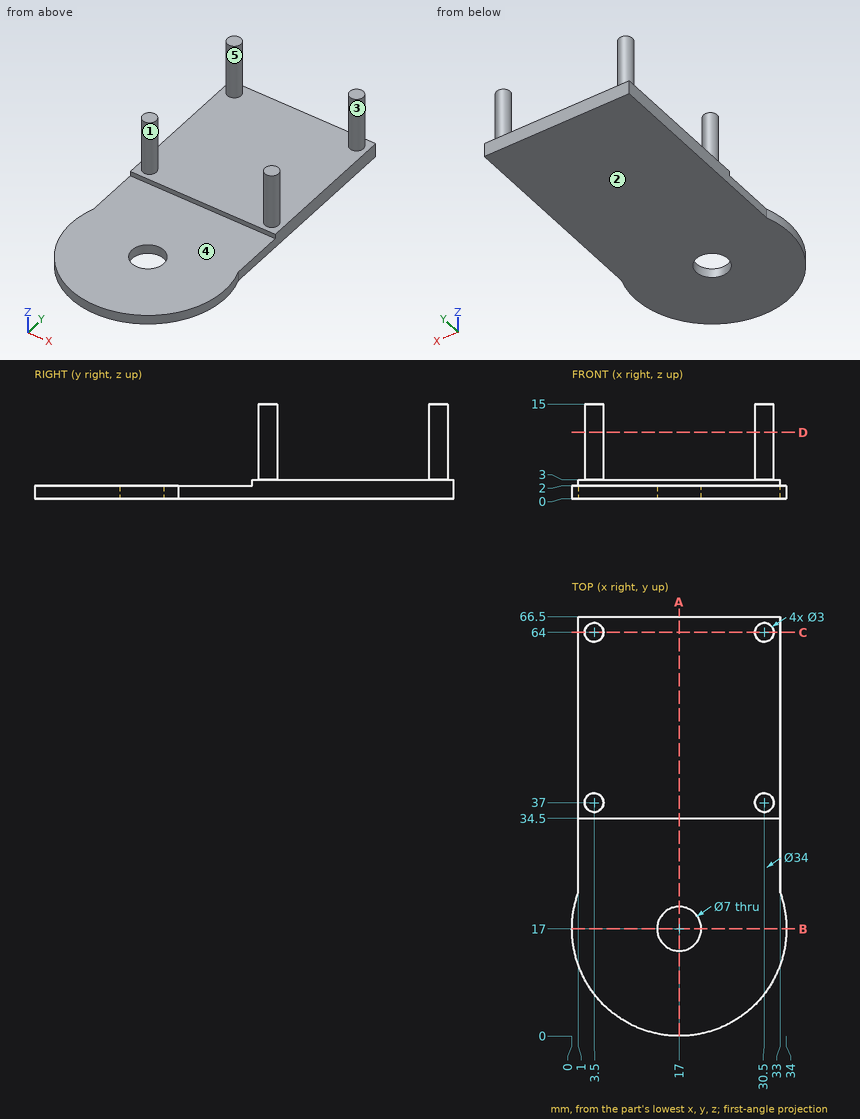
Input: dimensioned drawing with shaded views. Units: mm. Origin: part minimum x, y, z. A direction names the side the tool comes from. Coordinates: 2 decimals unless noted, no trailing zeros. Loops run counter-clockwise (first coordinate to the right, second up) from the corner with the lowest first, then second, coordinate; pieces in that order, holes last. Notation, with made-up numbers: (86, -35) -> (124, -35) arc R10 ccw to (124, -27) -> close; hole circle Ø7 at (85, 2.5). An arc over 180 degrees is marked (long way). Use a Markdown table: item, result. Add a question column.
(1) Pin query (flat end, axial travel): pin 1 Ø0.9 at (y, z) = (51.5, 1.5) entering from -X; pin 2 Ø6 at (x, y) = (22, 17) entering from +Z; pin 3 Ø8 at (x, y) = (18.5, 46.5) entering from -Z; pin 4 Ø3 at (x, y) = (22, 51.5) entering from +Z. Return the tip coordinate at first contact, or that it passes through.
(2) Section query A-A, the plane x = 17. Return loops of the section in (y, z).
(3) Section query B-B, the plane y = 17. Return loops of the section in (x, z), plus the area to 3 significant figures.
(4) Line query: line 1 along Y through (x, z) = (17, 1.4); line 2 along Z through (x, y) = (17.5, 31.5); line 3 along Z through (x, y) = (10.5, 49). Output: solid intervals per line, ascending.
(5) Section query D-D, the plane z = 10.5. Return loops of the section in (x, y).
(6) Access query for the marked faces 1 and 2. Directions: +Z, -Z, +X, -X, +Y, -Y. A direction counts if a zero-diameter tool reaches every point of the face in a straight line with its end or side. Return the directions, or none.
(7) Mould query, pull axis X, two halves, no side actions, for the marked faces 3, 4 and 5. Classes: pulls with the +X half, pulls with the -X half, needs draft (parallel to the pull), parting line crosses it, or undercut.
(8) Section query C-C, the plane y = 64. Return loops of the section in (x, z), plus the area to 3 significant figures.
Answer:
| question | item | result |
|---|---|---|
| 1 | pin 1 | stops at x = 1 |
| 1 | pin 2 | stops at z = 2 |
| 1 | pin 3 | stops at z = 0 |
| 1 | pin 4 | stops at z = 3 |
| 2 | outline | (0, 0) -> (13.5, 0) -> (13.5, 2) -> (0, 2) -> close; (20.5, 0) -> (66.5, 0) -> (66.5, 3) -> (34.5, 3) -> (34.5, 2) -> (20.5, 2) -> close |
| 3 | outline | (0, 0) -> (13.5, 0) -> (13.5, 2) -> (0, 2) -> close; (20.5, 0) -> (34, 0) -> (34, 2) -> (20.5, 2) -> close |
| 3 | area | 54.0 mm^2 |
| 4 | line 1 | y = 0 to 13.5, 20.5 to 66.5 |
| 4 | line 2 | z = 0 to 2 |
| 4 | line 3 | z = 0 to 3 |
| 5 | outline | circle Ø3 at (3.5, 37); circle Ø3 at (3.5, 64); circle Ø3 at (30.5, 37); circle Ø3 at (30.5, 64) |
| 6 | face 1 | +Z |
| 6 | face 2 | -Z, +X, -X, +Y, -Y |
| 7 | face 3 | undercut |
| 7 | face 4 | needs draft |
| 7 | face 5 | undercut |
| 8 | outline | (1, 0) -> (33, 0) -> (33, 3) -> (32, 3) -> (32, 15) -> (29, 15) -> (29, 3) -> (5, 3) -> (5, 15) -> (2, 15) -> (2, 3) -> (1, 3) -> close |
| 8 | area | 168 mm^2 |
